Model file for the job. Use its own axes, mm. A direction names the side the tool comes from. Give positions to 0.01 mm unless a question says otherwise; leave off trailing zeros. Loops run counter-clockwise (first coordinate to the right, second up) from the corner with the lowest first, then second, coordinate; pieces in that order, holes last. Notation, with made-up numbers: M 36,85 L 65,85 A25 cw 65,121 Z; hole C 89.5,87 d9. An arc over 180 degrees is marked long. Answer in a Markdown table with one row per item.
```python
from build123d import *

# Parameters (mm, degrees)
SKETCH001_R  = 2.6
PAD_DEPTH    = 6
PAD001_DEPTH = 1.6
SKETCH003_W  = 3.7771358599
SKETCH003_H  = 3.8
PAD002_DEPTH = 18.2


with BuildPart() as part:
    # Sketch001 → Pad (new body)
    with BuildSketch(Plane.YZ.offset(8.7)):
        with BuildLine():
            ThreePointArc((0, -6), (4.2426406871, -4.2426406871), (6, 0))
            Line((6, 18.2), (6, 0))
            ThreePointArc((6, 18.2), (4.2426406871, 22.4426406871), (0, 24.2))
            Line((0, 24.2), (-6, 24.2))
            ThreePointArc((-6, 24.2), (-7.4371881489, 9.1), (-6, -6))
            Line((0, -6), (-6, -6))
        make_face()
        Circle(SKETCH001_R, mode=Mode.SUBTRACT)
        with Locations((0, 18.2)):
            Circle(SKETCH001_R, mode=Mode.SUBTRACT)
    extrude(amount=PAD_DEPTH)

    # Sketch002 → Pad001 (join)
    with BuildSketch(Plane.YZ.offset(8.7)):
        with BuildLine():
            ThreePointArc((0, 12.2), (3.6774423219, 13.4590699257), (5.8114989668, 16.707860677))
            Line((6, 17.4420237293), (5.8114989668, 16.707860677))
            Line((6, 0.7579762707), (6, 17.4420237293))
            Line((5.8114989668, 1.492139323), (6, 0.7579762707))
            ThreePointArc((5.8114989668, 1.492139323), (3.6774423219, 4.7409300743), (0, 6))
            Line((-7.3771358599, 6), (0, 6))
            ThreePointArc((-7.3771358599, 12.2), (-7.4371881489, 9.1), (-7.3771358599, 6))
            Line((0, 12.2), (-7.3771358599, 12.2))
        make_face()
    extrude(amount=-PAD001_DEPTH)

    # Sketch003 → Pad002 (join)
    with BuildSketch(Plane.YZ.offset(8.7)):
        with Locations((-4.2885679299, 9.1)):
            Rectangle(SKETCH003_W, SKETCH003_H)
    extrude(amount=-PAD002_DEPTH)


with BuildPart() as part_1:
    # Body004 placement: moved
    add(part.part.moved(Location((0, -72.6064407756, 0))))


solid = part_1.part
```
Q1. 3-axis set-ups, long thin cutter, end or side, ignore diameter. For faces 4 (the face through (8.7, -75, 20)), 5 (the face through (-1, -78.784, 9)), 6 (the face through (-1, -77, 7.2)): which of +Z, -Z, +X, -X, +Y, -Y reach the whole face in a straight line?
Reported:
| item | result |
|---|---|
| face 4 | +Z, -X, -Y |
| face 5 | +Z, -Z, -X, -Y |
| face 6 | -Z, -X, +Y, -Y |
Q2. Saw through at A-A (y = -76). Give the cut face in (x, z), and give its area (3 significant figures).
Reported:
| item | result |
|---|---|
| outline | M -9.5,7.2 L 7.1,7.2 L 7.1,6 L 8.7,6 L 8.7,-6 L 14.7,-6 L 14.7,24.2 L 8.7,24.2 L 8.7,12.2 L 7.1,12.2 L 7.1,11 L -9.5,11 Z |
| area | 254 mm² |
Q3. Mould opens along Z. For faces 1 (the face through (11.658, -75.204, 18.314)), 2 (the face through (12, -76, 24.2)), 3 (the face through (8, -76, 6)) say: released by +Z, released by -Z, zero draft, split by the parting line, or undercut.
Reported:
| item | result |
|---|---|
| face 1 | undercut |
| face 2 | released by +Z |
| face 3 | released by -Z |
Q4. Probe probe 1 along X at (y, z) = (-72.75, -4.5); probe 2 along Z at (x, y) = (2, -77.5); probe 3 along Y at (x, z) = (5, 9). List the from-to ranges inside material, lowest first.
Reported:
| item | result |
|---|---|
| probe 1 | 8.7 to 14.7 |
| probe 2 | 7.2 to 11 |
| probe 3 | -78.78 to -75.01 |
Q5. Saw through at C-C (x = 4.5). Give the cut face in (y, z), and give its area (3 significant figures).
Reported:
| item | result |
|---|---|
| outline | M -78.78,7.2 L -75.01,7.2 L -75.01,11 L -78.78,11 Z |
| area | 14.4 mm² |
Q6. Saw through at B-B (z = 20). Give the cut face in (x, y), and give its area (3 significant figures).
Reported:
| item | result |
|---|---|
| outline | M 8.7,-79.3 L 14.7,-79.3 L 14.7,-74.48 L 8.7,-74.48 Z; M 8.7,-70.73 L 14.7,-70.73 L 14.7,-66.88 L 8.7,-66.88 Z |
| area | 52.0 mm² |
Q7. Drop flat-ended pins along their axis: pin 1 (10 mm diameter, centred on x = -2, z = 2.5, fed in from +Y); pin 2 (1.9 mm diameter, centred on x = 0.5, y = -77, fed in from -Z); pin 3 (0.8 mm diameter, centred on x = 8, y = -76.5, fed in from -Z). Give the stop position or say it passes through.
Reported:
| item | result |
|---|---|
| pin 1 | y = -75.01 |
| pin 2 | z = 7.2 |
| pin 3 | z = 6 |
